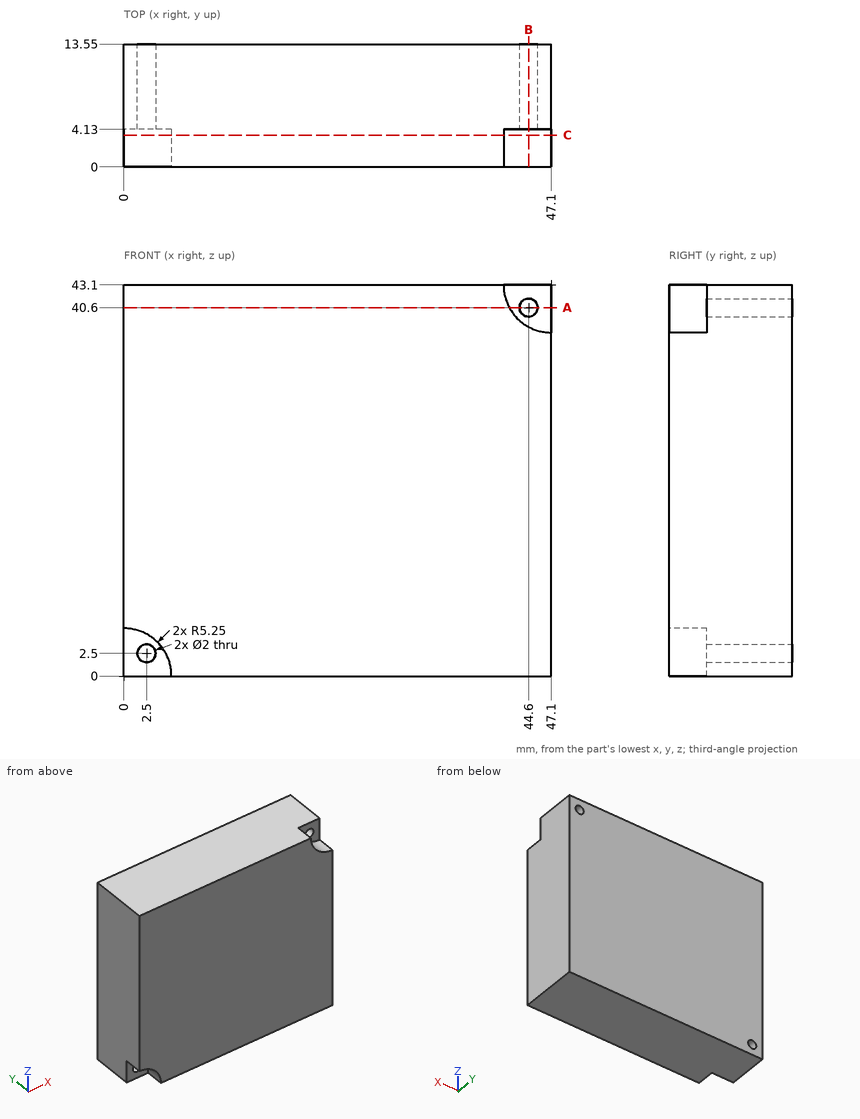
Could you check a few things on this drawing? It's one solid part, dimensions in mm from its lowest x, y, z. Round coordinates to 2 decimals unless told otherwise and drop trailing zeros. Loops run counter-clockwise (first coordinate to the right, second up) from the corner with the lowest first, then second, coordinate; pieces in that order, holes last. Notation, with made-up numbers: M -4.5,45 L 17.5,45 A18 ccw 17.5,51 Z; hole C -16,47.5 d3. An arc over 180 degrees is marked long. Write item = value, one per line. Start each with the question number.
(1) Suppose I cut it at B-B on x = 44.6. Write out the boundary of the cut face in (y, z).
(2) I need wall thicknesses on line 1 along Z through (x, y) = (44.6, 9.75); line 2 along Z through (x, y) = (2.5, 7); line 3 along X through (y, z) = (6.5, 41.5). Which ranges of each line are inside material? Lowest first, please.
(3) Suppose I cut it at A-A on z = 40.6. Write out the boundary of the cut face in (x, y), plus the area to 3 significant figures.
(4) Suppose I cut it at C-C on y = 3.5. Write out the boundary of the cut face in (x, z).
(5) I'm going to push a flat-ended pin straight in: P1, Ø2.5, axis at x = 2.5, z = 2.5, coming from the -Y side. Where does the tip first touch, or does it pass through?
Answer block:
q1.outline = M 0,0 L 13.55,0 L 13.55,39.6 L 4.13,39.6 L 4.13,38.48 L 0,38.48 Z; M 4.13,41.6 L 13.55,41.6 L 13.55,43.1 L 4.13,43.1 Z
q2.line_1 = 0 to 39.6, 41.6 to 43.1
q2.line_2 = 0 to 1.5, 3.5 to 43.1
q2.line_3 = 0 to 44.16, 45.04 to 47.1
q3.outline = M 0,0 L 42.48,0 L 42.48,4.13 L 43.6,4.13 L 43.6,13.55 L 0,13.55 Z; M 45.6,4.13 L 47.1,4.13 L 47.1,13.55 L 45.6,13.55 Z
q3.area = 600 mm²
q4.outline = M 0,5.25 A5.25 cw 5.25,0 L 47.1,0 L 47.1,37.85 A5.25 cw 41.85,43.1 L 0,43.1 Z
q5.P1 = 4.13
